Check sheet for the drawn part. Datum: minimum x, y, z corner. Units: mm. A direction names the side the tool comes from. Round coordinates to 2 decimals unless told otherwise and drop trailing zeros. Order: outer loops, then holes, each group sorted by start corner. A loop starts at its lowest first (then second) coordinate and runs counter-clockwise, first axis right, second up.
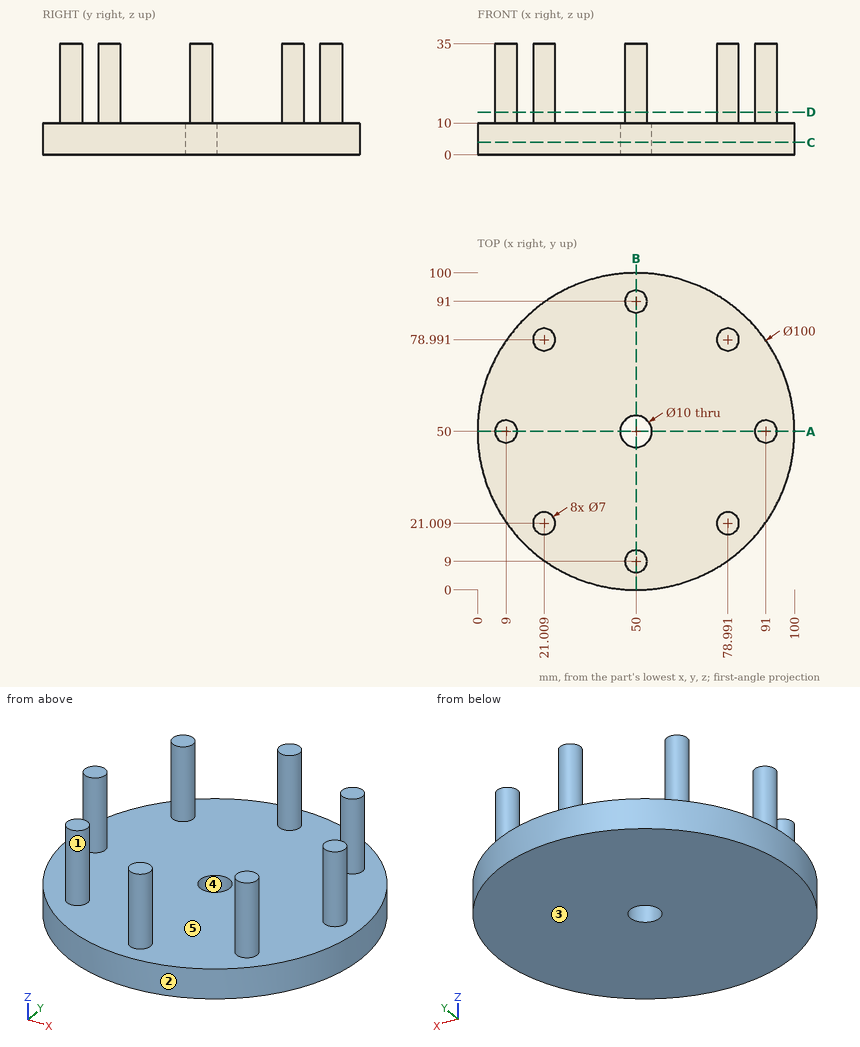
1) Sectioned sample at A-A on y = 50. Record the cut outline in (x, z), and give its area (3 significant figures).
2) Set-up check for the marked faces 4 and 5: record each of +Z, -Z, +X, -X, +Y, -Y from which the full face is reachable in a straight line by a thin tool's end or side.
3) Sectioned sample at D-D on z = 13.5. Record the cut outline in (x, y).
4) Gauge pin test, flat ends, axial feed: pin 1 (12 mm diameter, centred on y = 70.5, z = 30, fed in from +X); pin 2 (6 mm diameter, centred on x = 31, y = 63, fed in from +Z); pin 3 (8 mm diameter, centred on y = 77, z = 31, fed in from +X); pin 4 (3 mm diameter, centred on x = 49, y = 66.5, fed in from -Z). Record the tip position at first contact, or that the pin passes through.
5) Sectioned sample at C-C on z = 4. Record the cut outline in (x, y), and give its area (3 significant figures).
6) Draft check along Y on the marked faces 1, 2 and 3. Enter one of: pulls with the +Y half, pulls with the -Y half, needs draft (parallel to the pull), parting line crosses it, or undercut.
7) Scan lines: line 1 (Y direction, x = 50, z = 4.25); line 2 (Z direction, x = 27, y = 7); line 3 (Y direction, x = 52, z = 24.5). Record each from-to range of solid material in increasing order.
Values found:
1. outline: (0, 0) - (45, 0) - (45, 10) - (12.5, 10) - (12.5, 35) - (5.5, 35) - (5.5, 10) - (0, 10) - close; (55, 0) - (100, 0) - (100, 10) - (94.5, 10) - (94.5, 35) - (87.5, 35) - (87.5, 10) - (55, 10) - close
1. area: 1,250 mm2
2. face 4: +Z, -Z
2. face 5: +Z
3. outline: circle Ø7 at (9, 50); circle Ø7 at (21.01, 21.01); circle Ø7 at (21.01, 78.99); circle Ø7 at (50, 9); circle Ø7 at (50, 91); circle Ø7 at (78.99, 21.01); circle Ø7 at (78.99, 78.99); circle Ø7 at (91, 50)
4. pin 1: stops at x = 81.45
4. pin 2: stops at z = 10
4. pin 3: stops at x = 82.49
4. pin 4: stops at z = 0
5. outline: circle Ø100 at (50, 50); hole circle Ø10 at (50, 50)
5. area: 7,780 mm2
6. face 1: undercut
6. face 2: parting line crosses it
6. face 3: needs draft
7. line 1: y = 0 to 45, 55 to 100
7. line 2: z = 0 to 10
7. line 3: y = 6.13 to 11.87, 88.13 to 93.87
